```python
from build123d import *

# Parameters (mm, degrees)
F3_R     = 52
F4_DEPTH = 25.4
F5_DEPTH = 63.5


with BuildPart() as f2:
    # F0 (on Front) → F2 (revolve)
    with BuildSketch(Plane.XZ):
        with BuildLine():
            Line((54, 0), (0, 0))
            Line((0, 0), (0, -508))
            ThreePointArc((0, -508), (40.4620780602, -255.4310082977), (54, 0))
        make_face()
    revolve(axis=Axis((0, 0, 0), (0, 0, 1)))

    # F3 (on face) → F4 (join)
    with BuildSketch(Plane.XY):
        Circle(F3_R)
    extrude(amount=F4_DEPTH)

    # F5 (add): a face of the model
    f5_faces = [f2.faces().sort_by_distance(p)[0] for p in [
        (0, 0, 25.4),
    ]]
    extrude(f5_faces, amount=F5_DEPTH)


solid = f2.part
```
Geometry: final body of the model. Coordinates: model frame, mm. A direction names the side the tool comes from. Give positions to 0.01 mm unless a question says otherwise; leave off trailing zeros. Return JSON: item names as keys, results as strings.
Item 1: Line query: line 1 (X direction, y = 14, z = -14); line 2 (X direction, y = 2, z = -98); line 3 (Y direction, x = 21, z = -48.5). Output: solid intervals per line, ascending.
Filled in:
{"line 1": "-52.11 to 52.11", "line 2": "-51.97 to 51.97", "line 3": "-49.22 to 49.22"}
Item 2: Access query for faces 1 (the flat face through (-1, 1, 88.9)), 2 (the flat face through (-28, 44, 0)). Directions: +Z, -Z, +X, -X, +Y, -Y. A direction counts if a zero-diameter tool reaches every point of the face in a straight line with its end or side. Return the directions, or none.
Filled in:
{"face 1": "+Z, +X, -X, +Y, -Y", "face 2": "+Z"}
Item 3: Pin query (flat end, axial travel): P1, Ø5, axis at x = -10, z = -395.5, coming from the -Y side; P2, Ø10, axis at y = -38.5, z = -52.5, coming from the -X side; P3, Ø6, axis at y = 29, z = -290, coming from the +X side. Return the tip coordinate at first contact, or that it passes through.
Filled in:
{"P1": "y = -20.16", "P2": "x = -41.63", "P3": "x = 25.71"}
